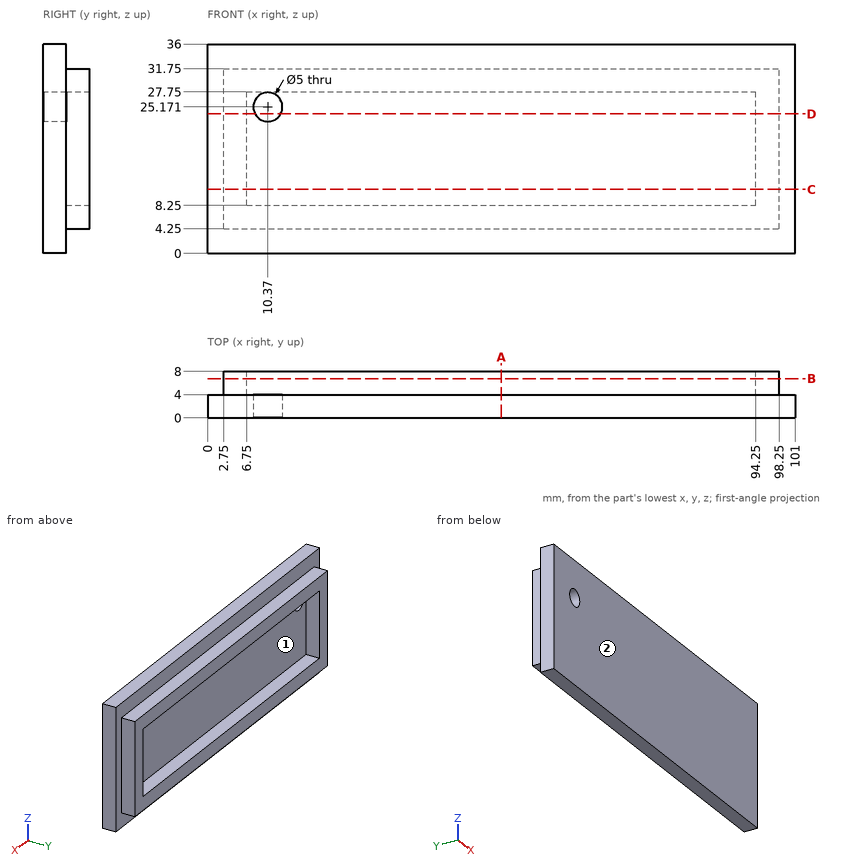
Geometry: see drawing. Coordinates: mm, zero at the bounding-box minimum. Round coordinates to 2 decimals unless told otherwise and drop trailing zeros. Write each loop counter-clockwise with the first axis right and the second up, starting at its lowest first coordinate (ties: lowest second). Pieces come first, ordered by that corner, then holes.
Item 1: Material intervals for L1, parallel to X at y = 4.25, z = 10.5; L2, parallel to Z at x = 52, y = 7; L3, parallel to X at y = 2.5, z = 25.5, sorted ascending.
Item 2: Section query D-D (z = 24). Return loops of the section in (x, y).
Item 3: Section query B-B (y = 6.75). Return loops of the section in (x, z), plus the area to 3 significant figures.
Item 4: Mould query, pull axis Z, two halves, no side actions, for the marked faces 1 and 2. Classes: +Z half, -Z half, draft (parallel to the pull), parting line (faces both ways), or undercut.
Item 5: Pin query (flat end, axial travel): P1, Ø1, axis at y = 7, z = 9, coming from the -X side; P2, Ø3, axis at x = 54, y = 7, coming from the -Z side; P3, Ø3, axis at x = 51, z = 13, coming from the -Y side; P4, Ø2, axis at x = 28.5, y = 6.5, coming from the +Z side. Return the tip coordinate at first contact, or that it passes through.
Item 6: Section query A-A (x = 50.5). Return loops of the section in (y, z).
Item 7: Section query C-C (z = 11). Return loops of the section in (x, y), plus the area to 3 significant figures.
Completed:
1. L1: x = 2.75 to 6.75, 94.25 to 98.25
1. L2: z = 4.25 to 8.25, 27.75 to 31.75
1. L3: x = 0 to 7.89, 12.85 to 101
2. outline: (0, 0) - (8.16, 0) - (8.16, 4) - (6.75, 4) - (6.75, 8) - (2.75, 8) - (2.75, 4) - (0, 4) - close; (12.58, 0) - (101, 0) - (101, 4) - (98.25, 4) - (98.25, 8) - (94.25, 8) - (94.25, 4) - (12.58, 4) - close
3. outline: (2.75, 4.25) - (98.25, 4.25) - (98.25, 31.75) - (2.75, 31.75) - close; hole (6.75, 8.25) - (94.25, 8.25) - (94.25, 27.75) - (6.75, 27.75) - close
3. area: 920 mm2
4. face 1: undercut
4. face 2: draft
5. P1: stops at x = 2.75
5. P2: stops at z = 4.25
5. P3: stops at y = 0
5. P4: stops at z = 31.75
6. outline: (0, 0) - (4, 0) - (4, 4.25) - (8, 4.25) - (8, 8.25) - (4, 8.25) - (4, 27.75) - (8, 27.75) - (8, 31.75) - (4, 31.75) - (4, 36) - (0, 36) - close
7. outline: (0, 0) - (101, 0) - (101, 4) - (98.25, 4) - (98.25, 8) - (94.25, 8) - (94.25, 4) - (6.75, 4) - (6.75, 8) - (2.75, 8) - (2.75, 4) - (0, 4) - close
7. area: 436 mm2
